Could you check a few things on this drawing? It's one solid part, dimensions in mm from its lowest x, y, z. Round coordinates to 2 decimals unless told otherwise and drop trailing zeros. Order: outer loops, then holes, each group sorted by start corner. A loop starts at its lowest first (then second) coordinate and runs counter-clockwise, first axis right, second up.
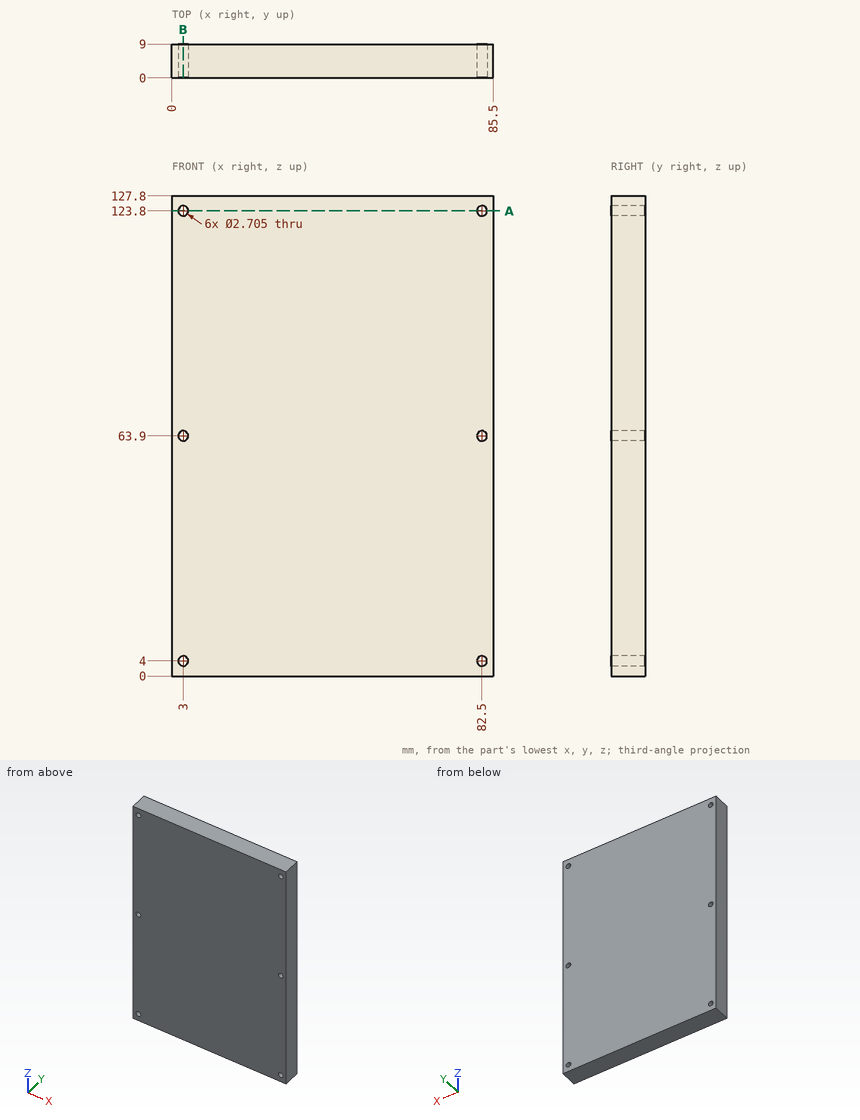
(1) Please list where these lines run through material, in increasing order: probe 1 along Z at (x, y) = (82.5, 2.5); probe 2 along X at (y, z) = (2.75, 123.8).
(2) I want a section at B-B, the plane x = 3. List the corners of the cut face in (y, z) for me.
(3) I'm going to push a flat-ended pin straight in: pin 1 Ø2.5 at (x, z) = (3, 4) entering from -Y. Where does the tip first touch, or does it pass through?
(4) I want a section at A-A, the plane z = 123.8. List the corners of the cut face in (x, y) for me, plus the area to 3 significant figures.
Ans:
1. probe 1: z = 0 to 2.65, 5.35 to 62.55, 65.25 to 122.45, 125.15 to 127.8
1. probe 2: x = 0 to 1.65, 4.35 to 81.15, 83.85 to 85.5
2. outline: (0, 0) - (9, 0) - (9, 2.65) - (0, 2.65) - close; (0, 5.35) - (9, 5.35) - (9, 62.55) - (0, 62.55) - close; (0, 65.25) - (9, 65.25) - (9, 122.45) - (0, 122.45) - close; (0, 125.15) - (9, 125.15) - (9, 127.8) - (0, 127.8) - close
3. pin 1: passes through
4. outline: (0, 0) - (1.65, 0) - (1.65, 9) - (0, 9) - close; (4.35, 0) - (81.15, 0) - (81.15, 9) - (4.35, 9) - close; (83.85, 0) - (85.5, 0) - (85.5, 9) - (83.85, 9) - close
4. area: 721 mm2
